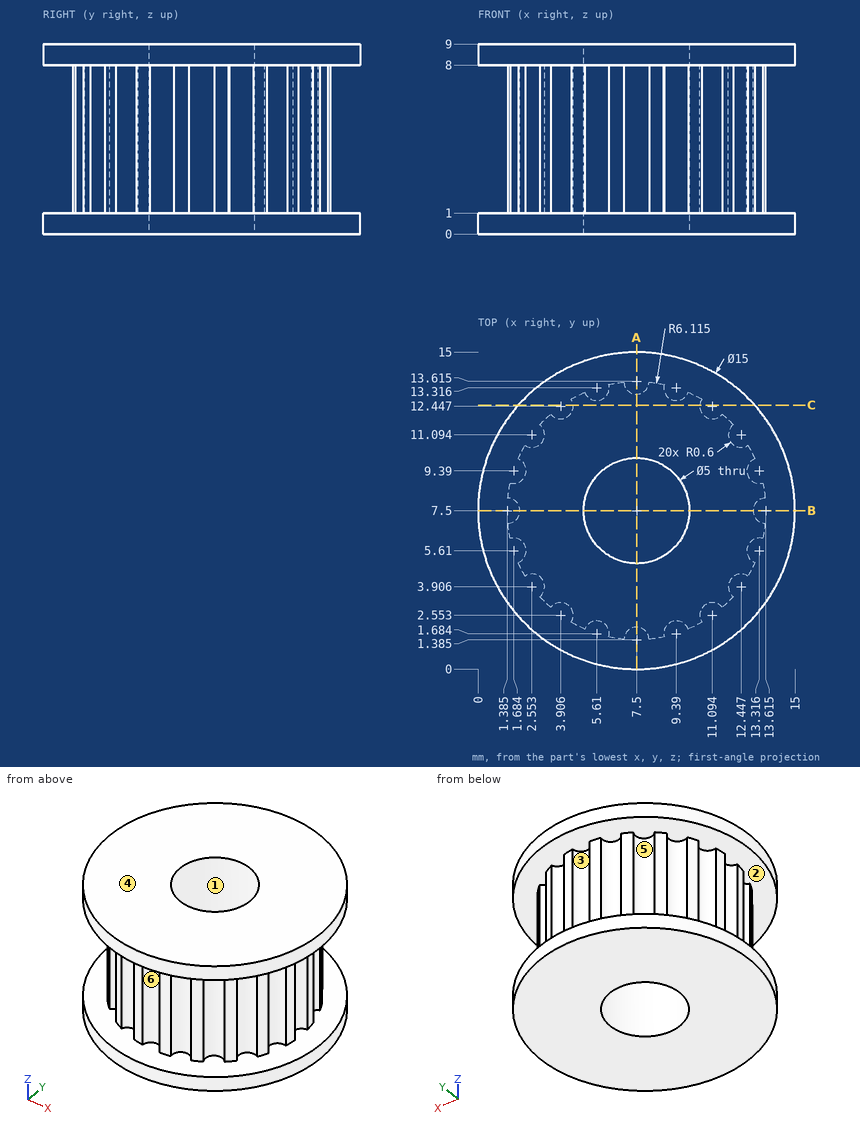
Drawing for the job (mm, zero at the part's lowest x, y, z). A direction names the side the tool comes from. Round coordinates to 2 decimals unless told otherwise and drop trailing zeros. Write each loop counter-clockwise with the first axis right and the second up, starting at its lowest first coordinate (ties: lowest second). Pieces come first, ordered by that corner, then holes. Notation, with made-up numbers: M 25.25,2.25 L 70.25,2.25 A8 cw 70.25,13.25 Z; hole C -7,63.25 d11. An arc over 180 degrees is marked long. Put each result on its own line as item: value.
Item 1: Mould opens along Y. For the marked faces 4, 5 and 6 say: +Y half, -Y half, draft (parallel to the pull), parting line (faces both ways), or undercut.
Responses:
face 4: draft
face 5: undercut
face 6: -Y half
Item 2: Cut at A-A (x = 7.5). List the corners of the cut face in (y, z) (1 decimal).
Responses:
outline: M 0,0 L 5,0 L 5,9 L 0,9 L 0,8 L 2,8 L 2,1 L 0,1 Z; M 10,0 L 15,0 L 15,1 L 13,1 L 13,8 L 15,8 L 15,9 L 10,9 Z
Item 3: Probe L1, parallel to Y at x = 7.5, z = 2.25 (1 decimal); L2, parallel to Z at x = 3, y = 13; L3, parallel to X at y = 2.5, z = 3. List the from-to ranges inside material, lowest first. Write a range as from..to.
Responses:
L1: 2..5, 10..13
L2: 0..1, 8..9
L3: 4.5..10.5
Item 4: Cut at C-C (y = 12.5). List the corners of the cut face in (x, z).
Responses:
outline: M 1.91,0 L 13.09,0 L 13.09,1 L 10.5,1 L 10.5,8 L 13.09,8 L 13.09,9 L 1.91,9 L 1.91,8 L 4.5,8 L 4.5,1 L 1.91,1 Z
Item 5: Tool access for the marked faces 1, 2 and 3: list every direction of +Z, -Z, +X, -X, +Y, -Y with a clear straight run to the whole face (end or side of a thin tool).
Responses:
face 1: +Z, -Z
face 2: none
face 3: +Y
Item 6: Flat gauge pins, fed straight in: P1, Ø2, axis at x = 1.5, z = 5.5, coming from the -Y side; P2, Ø1, axis at y = 4.5, z = 6.5, coming from the +X side; P3, Ø2, axis at x = 13.5, z = 1, coming from the -Y side. Where does each tip first touch, or does it go through?
Responses:
P1: y = 4.41
P2: x = 13.08
P3: y = 1.91
